from build123d import *

# Parameters (mm, degrees)
SKETCH1_R        = 11
SKETCH1_R_2      = 9.5
OUTER_RING_DEPTH = 7
SKETCH2_R        = 6
SKETCH2_R_2      = 4
INNER_RING_DEPTH = 7
SKETCH3_R        = 9.5
SKETCH3_R_2      = 6
SHIELDS_DEPTH    = 6.4


with BuildPart() as part:
    # Sketch1 → Outer_ring (new body)
    with BuildSketch(Plane.XY):
        Circle(SKETCH1_R)
        Circle(SKETCH1_R_2, mode=Mode.SUBTRACT)
    extrude(amount=OUTER_RING_DEPTH)



with BuildPart() as body_2:
    # Sketch2 → Inner_ring (new body)
    with BuildSketch(Plane.XY):
        Circle(SKETCH2_R)
        Circle(SKETCH2_R_2, mode=Mode.SUBTRACT)
    extrude(amount=INNER_RING_DEPTH)


with BuildPart() as part_1:
    add(part.part)

    add(body_2.part)  # Shields merges body 2
    # Sketch3 → Shields (add)
    with BuildSketch(Plane.XY.offset(0.3)):
        Circle(SKETCH3_R)
        Circle(SKETCH3_R_2, mode=Mode.SUBTRACT)
    extrude(amount=SHIELDS_DEPTH)


solid = part_1.part
Work out the finished part from the listing and answer in its coordinate system (mm). A direction names the side the tool comes from. Round coordinates to 2 decimals unless told otherwise and drop trailing zeros. Write each loop counter-clockwise with the first axis right and the second up, starting at its lowest first coordinate (ties: lowest second). Pieces come first, ordered by that corner, then holes.
1) A cutting plane is placed at C-C (z = 3). Give the vertices of the cut face in (x, y), plus the area to 3 significant figures.
2) A cutting plane is placed at A-A (x = 0). Give the vertices of the cut face in (y, z).
3) A cutting plane is placed at B-B (y = -1). Give the vertices of the cut face in (x, z).
4) Given pin 1 Ø1.5 at (x, z) = (5, 2.5) entering from -Y; pin 2 Ø1.5 at (y, z) = (-4, 2) entering from +X; pin 3 Ø1.5 at (x, z) = (5.5, 1) entering from +Y, each flat-ended and moving along its own axis, determine where each tip first touches the part or whether it passes through.
5) The mould has two halves that part along X. Classify faces 1 (the cylindrical face through (-2.38, -10.74, 3.45)), 2 (the flat face through (-0.1, -6.2, 6.7)), 3 (the flat face through (-10, 0, 7)): pulls with the +X half, pulls with the -X half, needs draft (parallel to the pull), parting line crosses it, or undercut.
6) A cutting plane is placed at D-D (y = 9). Give the vertices of the cut face in (x, z), plus the area to 3 significant figures.
7) A tool of negligible diameter and unlimited length cuts with its end or side. For faces 4 (the cylindrical face through (-4.76, -3.65, 6.85)), 5 (the flat face through (-10, 0, 0)), 6 (the flat face through (-0.1, -6.2, 0.3)), from which of +Z, -Z, +X, -X, +Y, -Y can it reach the whole face along a straight path? Write none if from no direction.
8) Straight lines are drawn through the part: line 1 (Y direction, x = 0, z = 6.85); line 2 (Z direction, x = -0.5, y = 6.5); line 3 (Y direction, x = 3.5, z = 5.5). For each, find the intervals that lie inside material, in ascending order.
Completed:
1. outline: circle Ø22 at (0, 0); hole circle Ø8 at (0, 0)
1. area: 330 mm2
2. outline: (-11, 0) - (-9.5, 0) - (-9.5, 0.3) - (-6, 0.3) - (-6, 0) - (-4, 0) - (-4, 7) - (-6, 7) - (-6, 6.7) - (-9.5, 6.7) - (-9.5, 7) - (-11, 7) - close; (4, 0) - (6, 0) - (6, 0.3) - (9.5, 0.3) - (9.5, 0) - (11, 0) - (11, 7) - (9.5, 7) - (9.5, 6.7) - (6, 6.7) - (6, 7) - (4, 7) - close
3. outline: (-10.95, 0) - (-9.45, 0) - (-9.45, 0.3) - (-5.92, 0.3) - (-5.92, 0) - (-3.87, 0) - (-3.87, 7) - (-5.92, 7) - (-5.92, 6.7) - (-9.45, 6.7) - (-9.45, 7) - (-10.95, 7) - close; (3.87, 0) - (5.92, 0) - (5.92, 0.3) - (9.45, 0.3) - (9.45, 0) - (10.95, 0) - (10.95, 7) - (9.45, 7) - (9.45, 6.7) - (5.92, 6.7) - (5.92, 7) - (3.87, 7) - close
4. pin 1: stops at y = -10.15
4. pin 2: stops at x = 10.51
4. pin 3: stops at y = 9.92
5. face 1: parting line crosses it
5. face 2: undercut
5. face 3: needs draft
6. outline: (-6.32, 0) - (-3.04, 0) - (-3.04, 0.3) - (3.04, 0.3) - (3.04, 0) - (6.32, 0) - (6.32, 7) - (3.04, 7) - (3.04, 6.7) - (-3.04, 6.7) - (-3.04, 7) - (-6.32, 7) - close
6. area: 84.9 mm2
7. face 4: +Z
7. face 5: -Z, +X, -X, +Y, -Y
7. face 6: -Z
8. line 1: y = -11 to -9.5, -6 to -4, 4 to 6, 9.5 to 11
8. line 2: z = 0.3 to 6.7
8. line 3: y = -10.43 to -1.94, 1.94 to 10.43
